```python
from build123d import *

# Parameters (mm, degrees)
F1_DEPTH     = 25.4
F2_T1_DEPTH  = 1.27
F2_T3_DEPTH  = 1.27
F2_T9_DEPTH  = 14.3341495789
F2_S10_R     = 3.81
F2_T11_DEPTH = 10
F2_T15_DEPTH = 14.3341495789
F2_S16_R     = 3.81
F2_T17_DEPTH = 10
F2_T24_DEPTH = 14.3341495789
F2_S25_R     = 3.81
F2_T26_DEPTH = 10
F2_T30_DEPTH = 14.3341495789
F2_S31_R     = 3.81
F2_T32_DEPTH = 10
F2_T39_DEPTH = 14.3341495789
F2_S40_R     = 3.81
F2_T41_DEPTH = 10
F2_T45_DEPTH = 14.3341495789
F2_S46_R     = 3.81
F2_T47_DEPTH = 10
F2_T54_DEPTH = 14.3341495789
F2_S55_R     = 3.81
F2_T56_DEPTH = 10
F2_T60_DEPTH = 14.3341495789
F2_S61_R     = 3.81
F2_T62_DEPTH = 10
F3_R         = 0.635


# Not quite as in the source:
# - a fillet or chamfer that OpenCascade refuses, or shapes differently, is made with other operations: its cross-section is extruded or revolved along the edge and cut away or added


with BuildPart() as f1:
    # F0 (on Top) → F1 (new body)
    with BuildSketch(Plane.XY):
        with BuildLine():
            ThreePointArc((3.7567106623, -0.635), (3.7966542918, -0.3186160517), (3.81, 0))
            ThreePointArc((3.81, 0), (3.7966542918, 0.3186160517), (3.7567106623, 0.635))
            Line((3.7567106623, 0.635), (0.635, 0.635))
            Line((0.635, 0.635), (0.635, -0.635))
            Line((0.635, -0.635), (3.7567106623, -0.635))
        make_face()
        with BuildLine():
            ThreePointArc((3.7567106623, 0.635), (3.7966542918, 0.3186160517), (3.81, 0))
            ThreePointArc((3.81, 0), (3.7966542918, -0.3186160517), (3.7567106623, -0.635))
            Line((3.7567106623, -0.635), (5.08, -0.635))
            Line((5.08, -0.635), (5.08, 0.635))
            Line((5.08, 0.635), (3.7567106623, 0.635))
        make_face()
        with BuildLine():
            Line((0.635, 0.635), (3.7567106623, 0.635))
            ThreePointArc((3.7567106623, 0.635), (2.6940768363, 2.6940768363), (0.635, 3.7567106623))
            Line((0.635, 3.7567106623), (0.635, 0.635))
        make_face()
        with BuildLine():
            ThreePointArc((0.635, -3.7567106623), (2.6940768363, -2.6940768363), (3.7567106623, -0.635))
            Line((3.7567106623, -0.635), (0.635, -0.635))
            Line((0.635, -0.635), (0.635, -3.7567106623))
        make_face()
        with BuildLine():
            Line((0.635, 0.635), (0.635, 3.7567106623))
            ThreePointArc((0.635, 3.7567106623), (0, 3.81), (-0.635, 3.7567106623))
            Line((-0.635, 3.7567106623), (-0.635, 0.635))
            Line((-0.635, 0.635), (0.635, 0.635))
        make_face()
        with BuildLine():
            ThreePointArc((-0.635, 3.7567106623), (0, 3.81), (0.635, 3.7567106623))
            Line((0.635, 3.7567106623), (0.635, 5.08))
            Line((0.635, 5.08), (-0.635, 5.08))
            Line((-0.635, 5.08), (-0.635, 3.7567106623))
        make_face()
        with BuildLine():
            Line((0.635, -5.08), (0.635, -3.7567106623))
            ThreePointArc((0.635, -3.7567106623), (0, -3.81), (-0.635, -3.7567106623))
            Line((-0.635, -3.7567106623), (-0.635, -5.08))
            Line((-0.635, -5.08), (0.635, -5.08))
        make_face()
        with BuildLine():
            ThreePointArc((-0.635, -3.7567106623), (0, -3.81), (0.635, -3.7567106623))
            Line((0.635, -3.7567106623), (0.635, -0.635))
            Line((0.635, -0.635), (-0.635, -0.635))
            Line((-0.635, -0.635), (-0.635, -3.7567106623))
        make_face()
        with BuildLine():
            Line((-0.635, 0.635), (-0.635, 3.7567106623))
            ThreePointArc((-0.635, 3.7567106623), (-2.6940768363, 2.6940768363), (-3.7567106623, 0.635))
            Line((-3.7567106623, 0.635), (-0.635, 0.635))
        make_face()
        with BuildLine():
            Line((-0.635, -0.635), (-0.635, 0.635))
            Line((-0.635, 0.635), (-3.7567106623, 0.635))
            ThreePointArc((-3.7567106623, 0.635), (-3.81, 0), (-3.7567106623, -0.635))
            Line((-3.7567106623, -0.635), (-0.635, -0.635))
        make_face()
        with BuildLine():
            ThreePointArc((-3.7567106623, -0.635), (-2.6940768363, -2.6940768363), (-0.635, -3.7567106623))
            Line((-0.635, -3.7567106623), (-0.635, -0.635))
            Line((-0.635, -0.635), (-3.7567106623, -0.635))
        make_face()
        with BuildLine():
            ThreePointArc((-3.7567106623, -0.635), (-3.81, 0), (-3.7567106623, 0.635))
            Line((-3.7567106623, 0.635), (-5.08, 0.635))
            Line((-5.08, 0.635), (-5.08, -0.635))
            Line((-5.08, -0.635), (-3.7567106623, -0.635))
        make_face()
    extrude(amount=F1_DEPTH)

    # F2: chamfer of 5.08 on 4 edges, made by hand

    # F2_s2 → F2_t1 (cut)
    with BuildSketch(Plane.YZ.offset(-0.635)):
        Polygon((0.635, 20.32), (5.715, 25.4), (0.635, 25.4), align=None)
        Polygon((-0.635, 20.32), (-5.715, 25.4), (-0.635, 25.4), align=None)
    extrude(amount=F2_T1_DEPTH, mode=Mode.SUBTRACT)

    # F2_s4 → F2_t3 (cut)
    with BuildSketch(Plane.XZ.offset(-0.635)):
        Polygon((-0.635, 20.32), (-5.715, 25.4), (-0.635, 25.4), align=None)
        Polygon((0.635, 20.32), (5.715, 25.4), (0.635, 25.4), align=None)
    extrude(amount=F2_T3_DEPTH, mode=Mode.SUBTRACT)


with BuildPart() as f2_tool7:
    # F2_s8 → F2_t9 (new body)
    with BuildSketch(Plane.XZ.offset(0.635)):
        Polygon((-0.635, 20.32), (-5.715, 25.4), (-0.635, 25.4), align=None)
    extrude(amount=-F2_T9_DEPTH)

    # F2_s10 → F2_t11 (intersect, symmetric)
    with BuildSketch(Plane.XY.offset(22.9)):
        Circle(F2_S10_R)
    extrude(amount=F2_T11_DEPTH, both=True, mode=Mode.INTERSECT)

    split(bisect_by=Plane.XZ.offset(-0.635), keep=Keep.BOTTOM)


with BuildPart() as f2_tool13:
    # F2_s14 → F2_t15 (new body)
    with BuildSketch(Plane.YZ.offset(-13.6991495789)):
        Polygon((0.635, 20.32), (5.715, 25.4), (0.635, 25.4), align=None)
    extrude(amount=F2_T15_DEPTH)

    # F2_s16 → F2_t17 (intersect, symmetric)
    with BuildSketch(Plane.XY.offset(22.9)):
        Circle(F2_S16_R)
    extrude(amount=F2_T17_DEPTH, both=True, mode=Mode.INTERSECT)

    split(bisect_by=Plane.YZ.offset(-0.635), keep=Keep.BOTTOM)


with BuildPart() as f2_tool7_1:
    add(f2_tool7.part)

    # F2_t19: intersect F2_tool13
    add(f2_tool13.part, mode=Mode.INTERSECT)


with BuildPart() as f1_1:
    add(f1.part)

    # F2_t5: cut F2_tool7
    add(f2_tool7_1.part, mode=Mode.SUBTRACT)


with BuildPart() as f2_tool22:
    # F2_s23 → F2_t24 (new body)
    with BuildSketch(Plane.YZ.offset(-0.635)):
        Polygon((0.635, 20.32), (5.715, 25.4), (0.635, 25.4), align=None)
    extrude(amount=F2_T24_DEPTH)

    # F2_s25 → F2_t26 (intersect, symmetric)
    with BuildSketch(Plane.XY.offset(22.9)):
        Circle(F2_S25_R)
    extrude(amount=F2_T26_DEPTH, both=True, mode=Mode.INTERSECT)

    split(bisect_by=Plane.YZ.offset(0.635), keep=Keep.TOP)


with BuildPart() as f2_tool28:
    # F2_s29 → F2_t30 (new body)
    with BuildSketch(Plane.XZ.offset(-13.6991495789)):
        Polygon((0.635, 20.32), (5.715, 25.4), (0.635, 25.4), align=None)
    extrude(amount=F2_T30_DEPTH)

    # F2_s31 → F2_t32 (intersect, symmetric)
    with BuildSketch(Plane.XY.offset(22.9)):
        Circle(F2_S31_R)
    extrude(amount=F2_T32_DEPTH, both=True, mode=Mode.INTERSECT)

    split(bisect_by=Plane.XZ.offset(-0.635), keep=Keep.BOTTOM)


with BuildPart() as f2_tool22_1:
    add(f2_tool22.part)

    # F2_t34: intersect F2_tool28
    add(f2_tool28.part, mode=Mode.INTERSECT)


with BuildPart() as f1_2:
    add(f1_1.part)

    # F2_t20: cut F2_tool22
    add(f2_tool22_1.part, mode=Mode.SUBTRACT)


with BuildPart() as f2_tool37:
    # F2_s38 → F2_t39 (new body)
    with BuildSketch(Plane.YZ.offset(0.635)):
        Polygon((-0.635, 20.32), (-5.715, 25.4), (-0.635, 25.4), align=None)
    extrude(amount=-F2_T39_DEPTH)

    # F2_s40 → F2_t41 (intersect, symmetric)
    with BuildSketch(Plane.XY.offset(22.9)):
        Circle(F2_S40_R)
    extrude(amount=F2_T41_DEPTH, both=True, mode=Mode.INTERSECT)

    split(bisect_by=Plane.YZ.offset(-0.635), keep=Keep.BOTTOM)


with BuildPart() as f2_tool43:
    # F2_s44 → F2_t45 (new body)
    with BuildSketch(Plane.XZ.offset(13.6991495789)):
        Polygon((-0.635, 20.32), (-5.715, 25.4), (-0.635, 25.4), align=None)
    extrude(amount=-F2_T45_DEPTH)

    # F2_s46 → F2_t47 (intersect, symmetric)
    with BuildSketch(Plane.XY.offset(22.9)):
        Circle(F2_S46_R)
    extrude(amount=F2_T47_DEPTH, both=True, mode=Mode.INTERSECT)

    split(bisect_by=Plane.XZ.offset(0.635), keep=Keep.TOP)


with BuildPart() as f2_tool37_1:
    add(f2_tool37.part)

    # F2_t49: intersect F2_tool43
    add(f2_tool43.part, mode=Mode.INTERSECT)


with BuildPart() as f1_3:
    add(f1_2.part)

    # F2_t35: cut F2_tool37
    add(f2_tool37_1.part, mode=Mode.SUBTRACT)


with BuildPart() as f2_tool52:
    # F2_s53 → F2_t54 (new body)
    with BuildSketch(Plane.YZ.offset(13.6991495789)):
        Polygon((-0.635, 20.32), (-5.715, 25.4), (-0.635, 25.4), align=None)
    extrude(amount=-F2_T54_DEPTH)

    # F2_s55 → F2_t56 (intersect, symmetric)
    with BuildSketch(Plane.XY.offset(22.9)):
        Circle(F2_S55_R)
    extrude(amount=F2_T56_DEPTH, both=True, mode=Mode.INTERSECT)

    split(bisect_by=Plane.YZ.offset(0.635), keep=Keep.TOP)


with BuildPart() as f2_tool58:
    # F2_s59 → F2_t60 (new body)
    with BuildSketch(Plane.XZ.offset(-0.635)):
        Polygon((0.635, 20.32), (5.715, 25.4), (0.635, 25.4), align=None)
    extrude(amount=F2_T60_DEPTH)

    # F2_s61 → F2_t62 (intersect, symmetric)
    with BuildSketch(Plane.XY.offset(22.9)):
        Circle(F2_S61_R)
    extrude(amount=F2_T62_DEPTH, both=True, mode=Mode.INTERSECT)

    split(bisect_by=Plane.XZ.offset(0.635), keep=Keep.TOP)


with BuildPart() as f2_tool52_1:
    add(f2_tool52.part)

    # F2_t64: intersect F2_tool58
    add(f2_tool58.part, mode=Mode.INTERSECT)


with BuildPart() as f1_4:
    add(f1_3.part)

    # F2_t50: cut F2_tool52
    add(f2_tool52_1.part, mode=Mode.SUBTRACT)

    # F3
    f3_edges = [f1_4.edges().sort_by_distance(p)[0] for p in [
        (5.08, 0, 24.765),
        (0, 5.08, 24.765),
        (-5.08, 0, 24.765),
        (0, -5.08, 24.765),
    ]]
    fillet(f3_edges, radius=F3_R)


solid = f1_4.part
```
Input: part model. Units: mm. Frame: model coordinates. A direction names the side the tool comes from. Round coordinates to 2 decimals unless told otherwise and drop trailing zeros. Loops run counter-clockwise (first coordinate to the right, second up) from the corner with the lowest first, then second, coordinate; pieces in that order, holes last. Notation, with made-up numbers: M 3,31 L 44,31 A24 ccw 44,48 Z; hole C 23,83 d10. An arc over 180 degrees is marked long. Answer in a Markdown table with one row per item. Add a question column.
1. Set-up query: faces 5 (the face through (0, -0.635, 10)), 6 (the face through (2.292, 0.038, 21.977)), 7 (the face through (-0.009, 4.698, 23.815)), 8 (the face through (-0.635, 4, 12)), 9 (the face through (4, 0.635, 12)). Return all of +Z, -Z, +X, -X, +Y, -Y with unobstructed straight access to the full face (end or side cutting, diameter ignored); none if empty.
2. Section A-A (x = 0). Output: boundary loops of the cut face in (y, z) (3 decimals).
3. Section B-B (z = 7.25). Output: boundary loops of the cut face in (x, y) (3 decimals), and give its area (3 significant figures).
4. Mould query, pull axis X, two halves, no side actions, for faces 1 (the face through (4.698, 0.009, 23.815)), 2 (the face through (4, -0.635, 12)), 3 (the face through (0.635, 0, 10)), 4 (the face through (0.635, -4, 12)). Classes: released by +X, released by -X, zero draft, split by the parting line, or undercut.
5. Section D-D (x = -1.5). Output: boundary loops of the cut face in (y, z) (3 decimals), and give its area (3 significant figures).
6. Contact query for flat-ended pins moving along their axis: pin 1 (2 mm diameter, centred on x = -4, z = 3, fed in from +Y); pin 2 (1.1 mm diameter, centred on y = -4.5, z = 15.5, fed in from +X) (3 decimals); pin 3 (0.7 mm diameter, centred on x = 4.5, z = 8.5, fed in from -Y) (3 decimals). Output: stop coordinate, or through.
7. Section C-C (y = 2). Output: boundary loops of the cut face in (x, z) (3 decimals).
8. Ray query, probe 1 along X at (y, z) = (4, 11.75) (3 decimals); probe 2 along X at (y, z) = (1, 7). Return the intervals inside material, ascending.
Values follow:
| question | item | result |
|---|---|---|
| 1 | face 5 | +Z, -Z |
| 1 | face 6 | +Z |
| 1 | face 7 | +Z, +X, -X |
| 1 | face 8 | +Z, -Z, -X, +Y |
| 1 | face 9 | +Z, -Z, +X, +Y |
| 2 | outline | M -5.08,0 L -0.635,0 L -0.635,20.32 L -3.996,23.681 A0.635 ccw -5.08,23.232 Z; M 0.635,0 L 5.08,0 L 5.08,23.232 A0.635 ccw 3.996,23.681 L 0.635,20.32 Z |
| 3 | outline | M -5.08,-0.635 L -3.757,-0.635 A3.81 ccw -0.635,-3.757 L -0.635,-5.08 L 0.635,-5.08 L 0.635,-3.757 A3.81 ccw 3.757,-0.635 L 5.08,-0.635 L 5.08,0.635 L 3.757,0.635 A3.81 ccw 0.635,3.757 L 0.635,5.08 L -0.635,5.08 L -0.635,3.757 A3.81 ccw -3.757,0.635 L -5.08,0.635 Z; hole M -0.635,-0.635 L 0.635,-0.635 L 0.635,0.635 L -0.635,0.635 Z |
| 3 | area | 50.5 mm^2 |
| 4 | face 1 | undercut |
| 4 | face 2 | zero draft |
| 4 | face 3 | undercut |
| 4 | face 4 | released by +X |
| 5 | outline | M -3.502,0 L 3.502,0 L 3.502,23.187 L 1.5,21.185 L -1.5,21.185 L -3.502,23.187 Z |
| 5 | area | 152 mm^2 |
| 6 | pin 1 | y = 2.35 |
| 6 | pin 2 | x = 0.635 |
| 6 | pin 3 | y = -0.635 |
| 7 | outline | M -3.243,0 L 3.243,0 L 3.243,22.928 L 2,21.685 L -2,21.685 L -3.243,22.928 Z |
| 8 | probe 1 | -0.635 to 0.635 |
| 8 | probe 2 | -3.68 to 3.68 |
